from build123d import *

# Parameters (mm, degrees)
SKETCH1_R                                           = 16
SKETCH1_R_2                                         = 10
BOSS_EXTRUDE1_DEPTH                                 = 34
SKETCH2_R                                           = 10
BOSS_EXTRUDE2_DEPTH                                 = 8
CBORE_FOR_M5_HEX_SOCKET_HEAD_CAP_SCREW1_D           = 5.5
CBORE_FOR_M5_HEX_SOCKET_HEAD_CAP_SCREW1_CBORE_D     = 9
CBORE_FOR_M5_HEX_SOCKET_HEAD_CAP_SCREW1_CBORE_DEPTH = 5.1
FILLET1_R                                           = 1


with BuildPart() as part:
    # Sketch1 → Boss-Extrude1 (new body)
    with BuildSketch(Plane.XY):
        Circle(SKETCH1_R)
        Circle(SKETCH1_R_2, mode=Mode.SUBTRACT)
    extrude(amount=BOSS_EXTRUDE1_DEPTH)

    # Sketch2 → Boss-Extrude2 (add)
    with BuildSketch(Plane.XY.offset(34)):
        with BuildLine():
            Line((-19.183326093, -19), (19.183326093, -19))
            ThreePointArc((19.183326093, -19), (27, 0), (19.183326093, 19))
            Line((19.183326093, 19), (-19.183326093, 19))
            ThreePointArc((-19.183326093, 19), (-27, 0), (-19.183326093, -19))
        make_face()
        Circle(SKETCH2_R, mode=Mode.SUBTRACT)
    extrude(amount=BOSS_EXTRUDE2_DEPTH)

    # CBORE for M5 Hex Socket Head Cap Screw1 (through all)
    with Locations(Plane(origin=(-18, -12, 42), x_dir=(1, 0, 0), z_dir=(0, 0, 1))):
        with Locations((0, 0), (0, 24), (36, 24), (36, 0)):
            CounterBoreHole(CBORE_FOR_M5_HEX_SOCKET_HEAD_CAP_SCREW1_D / 2, CBORE_FOR_M5_HEX_SOCKET_HEAD_CAP_SCREW1_CBORE_D / 2, CBORE_FOR_M5_HEX_SOCKET_HEAD_CAP_SCREW1_CBORE_DEPTH)

    # Fillet1
    fillet1_edges = [part.edges().sort_by_distance(p)[0] for p in [
        (-19.183326093, 19, 38),
        (-19.183326093, -19, 38),
        (19.183326093, -19, 38),
        (19.183326093, 19, 38),
    ]]
    fillet(fillet1_edges, radius=FILLET1_R)


solid = part.part
Build history of the part. All positions in model axes, mm. A direction names the side the tool comes from. Give positions to 0.01 mm unless a question says otherwise; leave off trailing zeros. Order: outer loops, then holes, each group sorted by start corner. A loop starts at its lowest first (then second) coordinate and runs counter-clockwise, first axis right, second up. Notation, with made-up numbers: M 12,52.25 L 17,52.25 A24 ccw 17,72.25 Z; hole C 46.5,61.5 d9. An arc over 180 degrees is marked long. Put each result on its own line as item: value.
Item 1: Two-plate mould, pull along X, no slides. Class faces 3 (the flat face through (6, 9, 42)), 4 (the flat face through (21, 12, 36.9)), 5 (the cylindrical face through (-3.47, -15.62, 16.76)), 6 (the cylindrical face through (27, 0, 38)): +X half, -X half, draft (parallel to the pull), parting line (faces both ways), or undercut.
From the geometry:
face 3: draft
face 4: undercut
face 5: parting line
face 6: +X half
Item 2: Slice it at B-B, the plane x = 18. Write the cut outline in (y, z).
From the geometry:
outline: M -19,34 L -14.75,34 L -14.75,36.9 L -16.5,36.9 L -16.5,42 L -19,42 Z; M -9.25,34 L 9.25,34 L 9.25,36.9 L 7.5,36.9 L 7.5,42 L -7.5,42 L -7.5,36.9 L -9.25,36.9 Z; M 14.75,34 L 19,34 L 19,42 L 16.5,42 L 16.5,36.9 L 14.75,36.9 Z
Item 3: Slice it at D-D, the plane z = 4. Write the cut outline in (x, y).
From the geometry:
outline: C 0,0 d32; hole C 0,0 d20
Item 4: Slice it at C-C, the plane y = -12. Write the cut outline in (x, z).
From the geometry:
outline: M -24.19,34 L -20.75,34 L -20.75,36.9 L -22.5,36.9 L -22.5,42 L -24.19,42 Z; M -15.25,34 L -10.58,34 L -10.58,0 L 10.58,0 L 10.58,34 L 15.25,34 L 15.25,36.9 L 13.5,36.9 L 13.5,42 L -13.5,42 L -13.5,36.9 L -15.25,36.9 Z; M 20.75,34 L 24.19,34 L 24.19,42 L 22.5,42 L 22.5,36.9 L 20.75,36.9 Z
Item 5: Slice it at A-A, the plane x = 0. Write the cut outline in (y, z).
From the geometry:
outline: M -19,34 L -16,34 L -16,0 L -10,0 L -10,42 L -19,42 Z; M 10,0 L 16,0 L 16,34 L 19,34 L 19,42 L 10,42 Z
Item 6: Flat gauge pins, fed straight in: pin 1 Ø8 at (x, y) = (-18, 12) entering from +Z; pin 2 Ø4 at (x, z) = (-5, 15.5) entering from -Y; pin 3 Ø8 at (x, z) = (-8, 8.5) entering from +Y; pin 4 Ø10 at (x, y) = (-17.5, -12.5) entering from +Z. Where does each tip first touch, or does it go through?
From the geometry:
pin 1: stops at z = 36.9
pin 2: stops at y = -15.72
pin 3: stops at y = 15.49
pin 4: stops at z = 42
Item 7: 3-axis set-ups, long thin cutter, end or side, ignore diameter. For faces 1 (the cylindrical face through (-15.253, -11.879, 35.43)), 2 (the flat face through (-15, -12, 36.9)): which of +Z, -Z, +X, -X, +Y, -Y reach the whole face in a straight line?
From the geometry:
face 1: +Z, -Z
face 2: +Z
Item 8: Probe line 1 (Y direction, x = -18, z = 34.8); line 2 (Y direction, x = -18, z = 40.5); line 3 (Z direction, x = -16, y = 1). List the from-to ranges inside material, lowest first. Write a range as [from, to].
From the geometry:
line 1: y = [-19, -14.75], [-9.25, 9.25], [14.75, 19]
line 2: y = [-19, -16.5], [-7.5, 7.5], [16.5, 19]
line 3: z = [34, 42]
